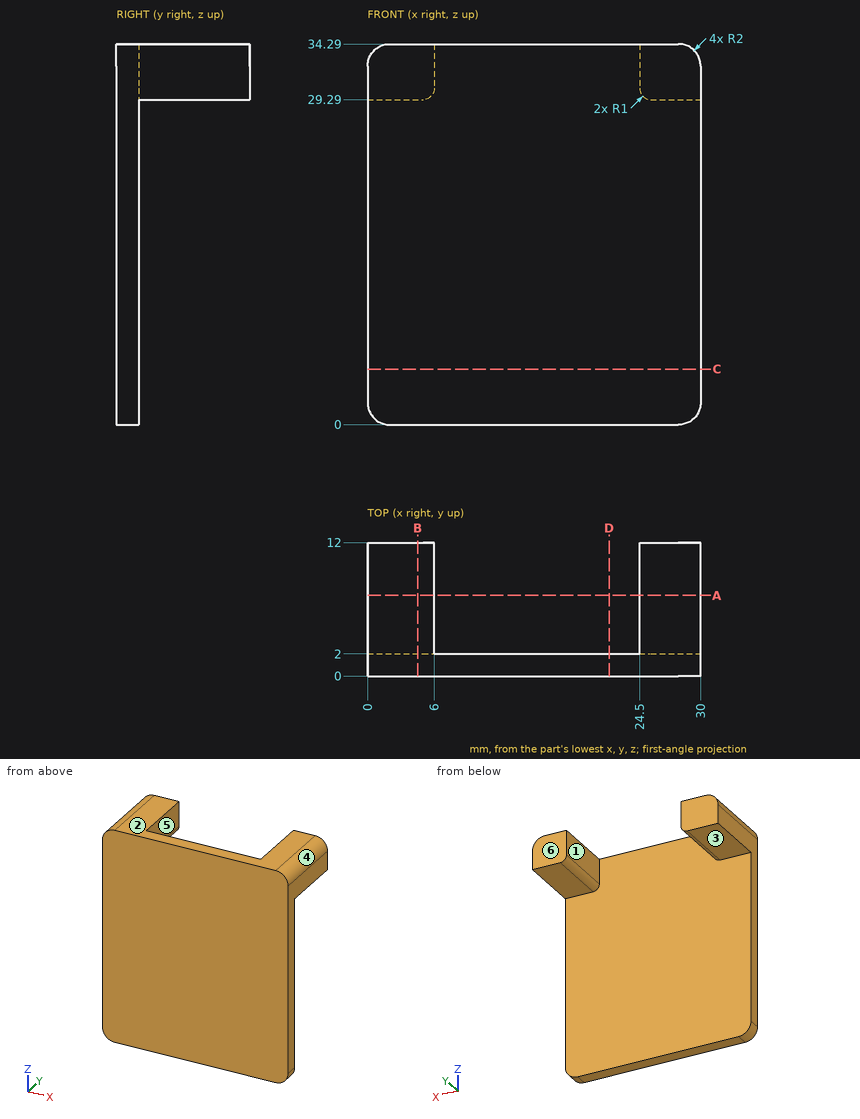
Job drawing, mm, ordinate dimensions from the low corner. One solid piece. A direction names the side the tool comes from. Coordinates: 2 decimals unless noted, no trailing zeros. Order: outer loops, then holes, each group sorted by start corner. A loop starts at its lowest first (then second) coordinate and runs counter-clockwise, first axis right, second up. Notation, with made-up numbers: (58.5, -11.5) -> (103.5, -11.5) arc R35 cw to (103.5, 21.5) -> close; hole circle Ø6 at (26, 38.5). An arc over 180 degrees is marked (long way). Answer in a Markdown table with one row per item. Add a question column.
Q1. Band-saw the part on D-D, the plane x = 21.75. List the corners of the cut face in (y, z), then the cut area to 3 significant figures.
Q2. Band-saw the part on A-A, the plane y = 7.25. List the corners of the cut face in (x, z), then the cut area to 3 significant figures.
Q3. Which spindle directions (+Z, -Z, +X, -X, +Y, -Y) get a long thin tool onto all of the face, cutting with end or side? Do the marked faces 1, 2 and 3. Say none if no direction does.
Q4. Band-saw the part on C-C, the plane z = 5. List the corners of the cut face in (x, y), then the cut area to 3 significant figures.
Q5. Mould opens along X. For the marked faces 4, 5 and 6 say: +X half, -X half, draft (parallel to the pull), parting line (faces both ways), or undercut.
Q6. Wall check: line 1 along X through (y, z) = (7.5, 32); line 2 along Y through (x, z) = (14, 11); line 3 along Z through (x, y) = (2, 2.25). Give the ranges that are in metal, low to high. Write a range as [from, to].
Q7. Drop flat-ended pins along their axis: pin 1 (1.5 mm diameter, centred on y = 7, z = 27, fed in from +X); pin 2 (12 mm diameter, centred on x = 12, z = 13.5, fed in from +Y); pin 3 (3 mm diameter, centred on x = 23.5, y = 6, fed in from -Z); pin 4 (3.5 mm diameter, centred on x = 28.5, y = 8.5, fed in from -Z). Give the stop position or say it passes through.
Q8. Band-saw the part on B-B, the plane x = 4.5. List the corners of the cut face in (y, z).
Answers follow:
| question | item | result |
|---|---|---|
| 1 | outline | (0, 0) -> (2, 0) -> (2, 34.29) -> (0, 34.29) -> close |
| 1 | area | 68.6 mm^2 |
| 2 | outline | (0, 29.29) -> (5, 29.29) arc R1 ccw to (6, 30.29) -> (6, 34.29) -> (2, 34.29) arc R2 ccw to (0, 32.29) -> close; (24.5, 30.29) arc R1 ccw to (25.5, 29.29) -> (30, 29.29) -> (30, 32.29) arc R2 ccw to (28, 34.29) -> (24.5, 34.29) -> close |
| 2 | area | 55.4 mm^2 |
| 3 | face 1 | +Z, -Z, +Y |
| 3 | face 2 | +Z, +X, -X, +Y, -Y |
| 3 | face 3 | -Z, +X, -X, +Y |
| 4 | outline | (0, 0) -> (30, 0) -> (30, 2) -> (0, 2) -> close |
| 4 | area | 60.0 mm^2 |
| 5 | face 4 | +X half |
| 5 | face 5 | undercut |
| 5 | face 6 | draft |
| 6 | line 1 | [0, 6], [24.5, 30] |
| 6 | line 2 | [0, 2] |
| 6 | line 3 | [29.29, 34.29] |
| 7 | pin 1 | through |
| 7 | pin 2 | y = 2 |
| 7 | pin 3 | z = 29.42 |
| 7 | pin 4 | z = 29.29 |
| 8 | outline | (0, 0) -> (2, 0) -> (2, 29.29) -> (12, 29.29) -> (12, 34.29) -> (0, 34.29) -> close |
